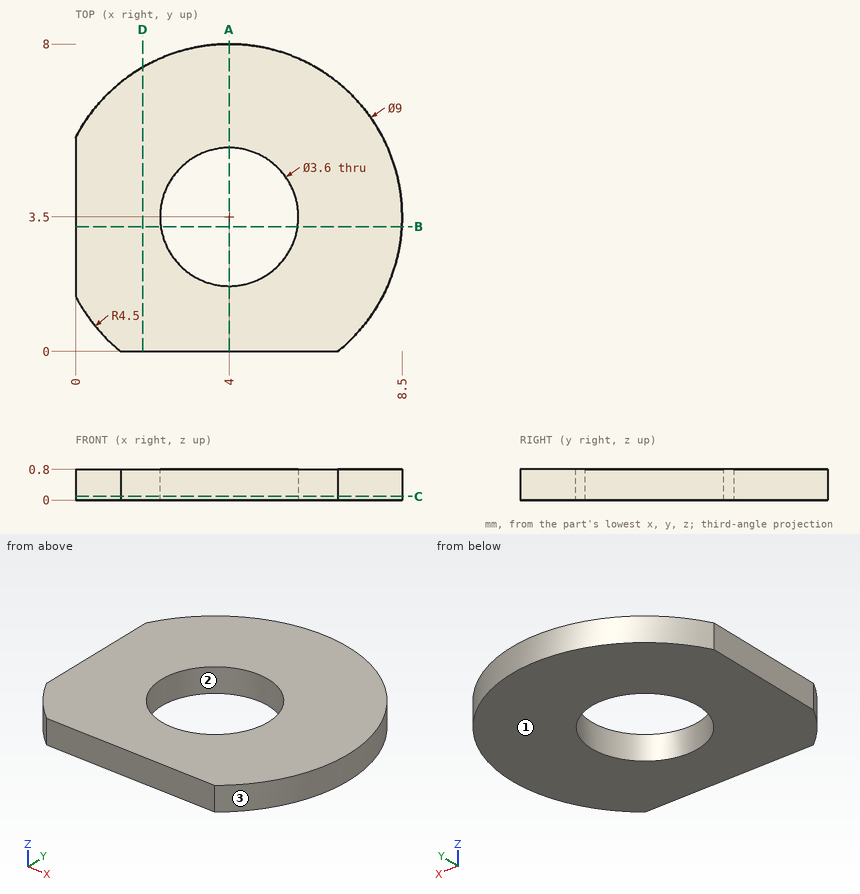
Check sheet for the drawn part. Datum: minimum x, y, z corner. Units: mm. Round coordinates to 2 decimals unless told otherwise and drop trailing zeros. Order: outer loops, then holes, each group sorted by start corner. A loop starts at its lowest first (then second) coordinate and runs counter-clockwise, first axis right, second up. Notation, with made-up numbers: (-18, 64) -> (0, 64) arc R26 ccw to (0, 97) -> close; hole circle Ø6 at (16.25, 79.5). An arc over 180 degrees is marked (long way). Put each result on its own line as item: value.
1) Section check A-A (x = 4). Record the cut outline in (y, z), then the cut area to 3 significant figures.
Final values:
outline: (0, 0) -> (1.7, 0) -> (1.7, 0.8) -> (0, 0.8) -> close; (5.3, 0) -> (8, 0) -> (8, 0.8) -> (5.3, 0.8) -> close
area: 3.52 mm^2
2) Section check C-C (z = 0.1). Record the cut outline in (x, y).
Final values:
outline: (0, 1.44) arc R4.5 ccw to (1.17, 0) -> (6.83, 0) arc R4.5 ccw (long way) to (0, 5.56) -> close; hole circle Ø3.6 at (4, 3.5)
3) Section check D-D (x = 1.75). Record the cut outline in (y, z), then the cut area to 3 significant figures.
Final values:
outline: (0, 0) -> (7.4, 0) -> (7.4, 0.8) -> (0, 0.8) -> close
area: 5.92 mm^2
4) Section check B-B (y = 3.25). Record the cut outline in (x, z), then the cut area to 3 significant figures.
Final values:
outline: (0, 0) -> (2.22, 0) -> (2.22, 0.8) -> (0, 0.8) -> close; (5.78, 0) -> (8.49, 0) -> (8.49, 0.8) -> (5.78, 0.8) -> close
area: 3.94 mm^2
5) Depth check by flat-ended pin: pin 1 (3 mm diameter, centred on x = 4, y = 3.5, fed in from -Z). Enter the tip coordinate at first touch or a pass-through.
Final values:
pin 1: passes through
6) Mould release check, pull along Y, two halves, no side actions. Record for the marked faces 1, 2 and 3: +Y half, -Y half, draft (parallel to the pull), parting line (faces both ways), or undercut.
Final values:
face 1: draft
face 2: undercut
face 3: parting line
7) Material ranges on line 1 (Y direction, x = 4, z = 0.4); line 2 (X direction, y = 3.5, z = 0.6); line 3 (Y direction, x = 4.5, z = 0.5), recorded low to high.
Final values:
line 1: y = 0 to 1.7, 5.3 to 8
line 2: x = 0 to 2.2, 5.8 to 8.5
line 3: y = 0 to 1.77, 5.23 to 7.97
